Work out the finished part from the listing and answer in its coordinate system (mm). Face numbers are marked on the shaded views. Coordinates: 2 decimals unless noted, no trailing zeros. Loops run counter-clockwise (first coordinate to the right, second up) from the corner with the lowest first, then second, coordinate; pieces in that order, holes last. Notation, with made-up numbers: (-1, 67.5) -> (37, 67.5) arc R18 cw to (37, 97.5) -> close; hole circle Ø9 at (65.5, 45). An arc over 180 degrees is marked (long way). Use a Markdown table: item, result.
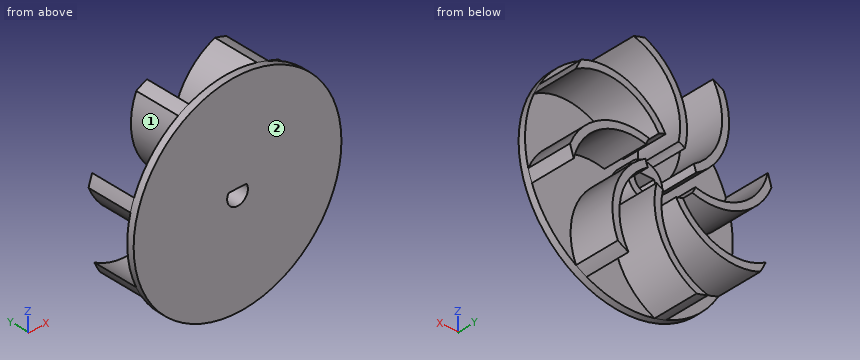
from build123d import *

# Parameters (mm, degrees)
SKETCH1_R           = 30
BOSS_EXTRUDE1_DEPTH = 2
SKETCH2_R           = 5
BOSS_EXTRUDE2_DEPTH = 7
BOSS_EXTRUDE3_DEPTH = 13
CUT_EXTRUDE1_DEPTH  = 16
CIRPATTERN2_COUNT   = 8


with BuildPart() as part:
    # Sketch1 → Boss-Extrude1 (new body)
    with BuildSketch(Plane(origin=(0, 0, 0), x_dir=(1, 0, 0), z_dir=(0, 1, 0))):
        Circle(SKETCH1_R)
    extrude(amount=BOSS_EXTRUDE1_DEPTH)

    # Sketch2 → Boss-Extrude2 (add)
    with BuildSketch(Plane(origin=(0, 0, 0), x_dir=(1, 0, 0), z_dir=(0, 1, 0))):
        Circle(SKETCH2_R)
    extrude(amount=BOSS_EXTRUDE2_DEPTH)

    # Sketch3 → Boss-Extrude3 (add)
    with BuildSketch(Plane(origin=(0, 2, 0), x_dir=(1, 0, 0), z_dir=(0, 1, 0))):
        with BuildLine():
            ThreePointArc((-1.505806951, 7.292266896), (-12.151790035, 15.86929072), (-25.810761164, 15.290670625))
            ThreePointArc((-25.810761164, 15.290670625), (-26.649690738, 13.776573724), (-27.399897799, 12.216611666))
            ThreePointArc((-27.399897799, 12.216611666), (-14.251932533, 14.383859932), (-3.429686075, 6.60922571))
            ThreePointArc((-3.429686075, 6.60922571), (-2.491266579, 7.016993793), (-1.505806951, 7.292266896))
        make_face()
    boss_extrude3 = extrude(amount=BOSS_EXTRUDE3_DEPTH)

    # Sketch4 → Cut-Extrude1 (cut, through all)
    with BuildSketch(Plane(origin=(0, 0, 0), x_dir=(1, 0, 0), z_dir=(0, 1, 0))):
        with BuildLine():
            Line((-2.598076211, -1.5), (2.598076211, -1.5))
            ThreePointArc((2.598076211, -1.5), (0, 3), (-2.598076211, -1.5))
        make_face()
    extrude(amount=CUT_EXTRUDE1_DEPTH, mode=Mode.SUBTRACT)

    # CirPattern2: Boss-Extrude3 ×8 about axis
    cirpattern2_axis = Axis((0, 0, 0), (0, 1, 0))
    for i in range(1, CIRPATTERN2_COUNT):
        add(boss_extrude3.rotate(cirpattern2_axis, i * 360 / CIRPATTERN2_COUNT))


solid = part.part
Q1. Section B-B on z = 0 is taken. Determine the outline of the cut face in (x, y), and give its area (3 significant figures).
Solved:
| item | result |
|---|---|
| outline | (-30, 0) -> (-3, 0) -> (-3, 7) -> (-5, 7) -> (-5, 2) -> (-20.4, 2) -> (-20.4, 15) -> (-23.74, 15) -> (-23.74, 2) -> (-30, 2) -> close; (3, 0) -> (30, 0) -> (30, 2) -> (23.74, 2) -> (23.74, 15) -> (20.4, 15) -> (20.4, 2) -> (5, 2) -> (5, 7) -> (3, 7) -> close |
| area | 215 mm² |
Q2. Section D-D on x = 13.5 is taken. Determine the outline of the cut face in (y, z), and give its area (3 significant figures).
Solved:
| item | result |
|---|---|
| outline | (0, -26.79) -> (15, -26.79) -> (15, -24.91) -> (2, -24.91) -> (2, -11.52) -> (15, -11.52) -> (15, -7.33) -> (2, -7.33) -> (2, 2.54) -> (15, 2.54) -> (15, 4.56) -> (2, 4.56) -> (2, 14.19) -> (15, 14.19) -> (15, 16.26) -> (2, 16.26) -> (2, 26.79) -> (0, 26.79) -> close |
| area | 239 mm² |
Q3. Given pin 1 Ø1.5 at (x, y) = (-6, 7.5) entering from +Z; pin 2 Ø9.5 at (x, z) = (0, 0) entering from +Y; pin 3 Ø6 at (y, z) = (12.5, 21.5) entering from +X, each flat-ended and moving along its own axis, determine where each tip first touches the part or whether it passes through.
Solved:
| item | result |
|---|---|
| pin 1 | z = 3.52 |
| pin 2 | y = 7 |
| pin 3 | x = 3.63 |
Q4. Determine the mould class of the marked faces 1 and 2 for opening direction X: pulls with the +X half, pulls with the -X half, needs draft (parallel to the pull), parting line crosses it, or undercut.
Solved:
| item | result |
|---|---|
| face 1 | undercut |
| face 2 | needs draft |
Q5. Consider line 1 (X direction, y = 1.5, z = 0); line 2 (Z direction, x = 0, y = 4.5); line 3 (Z direction, x = -7.5, y = 5.75). Determine where each line is inside the solid, lowest interval first. Write a range as [from, to].
Solved:
| item | result |
|---|---|
| line 1 | [-30, -3], [3, 30] |
| line 2 | [-23.74, -20.4], [-5, -3], [1.5, 5], [20.4, 23.74] |
| line 3 | [-29.05, -26.91], [-13.61, -11.15], [-4.38, -2.34], [1.63, 4.02] |
Q6. Section A-A on y = 12.5 is taken. State how many separate pieces and enclosed holes the cut face has, and give its area (3 significant figures).
Solved:
| item | result |
|---|---|
| separate pieces | 8 |
| enclosed holes | 0 |
| area | 442 mm² |
